Job drawing, mm, ordinate dimensions from the low corner. One solid piece. A direction names the side the tool comes from. Round coordinates to 2 decimals unless told otherwise and drop trailing zeros. Loops run counter-clockwise (first coordinate to the right, second up) from the corner with the lowest first, then second, coordinate; pieces in that order, holes last.
1) Mould opens along Z. For the marked faces 1, 2, 3 and 4 say: +Z half, -Z half, draft (parallel to the pull), parting line (faces both ways), or undercut.
2) Band-saw the part on B-B, the plane y = 5. Write the cut outline in (x, z), then the cut area to 3 significant figures.
3) Band-saw the part on C-C, the plane z = 2.25. Write the cut outline in (x, y).
4) Probe line 1 (Y direction, x = 7.5, z = 0.9); line 2 (X direction, y = 7, z = 12.25). List the from-to ranges inside material, lowest first.
5) Drop flat-ended pins along their axis: P1, Ø2, axis at y = 7.5, z = 5, coming from the +X side; P2, Ø2.5, axis at y = 5, z = 7.5, coming from the -X side. Give the stop position or say it passes through.
6) 3-axis set-ups, long thin cutter, end or side, ignore diameter. For the marked faces 5 and 6: which of +Z, -Z, +X, -X, +Y, -Y reach the whole face in a straight line?
7) Band-saw the part on D-D, the plane y = 9. Write the cut outline in (x, z), then the cut area to 3 significant figures.
8) Band-saw the part on A-A, the plane z = 7.5. Write the cut outline in (x, y), then the cut area to 3 significant figures.
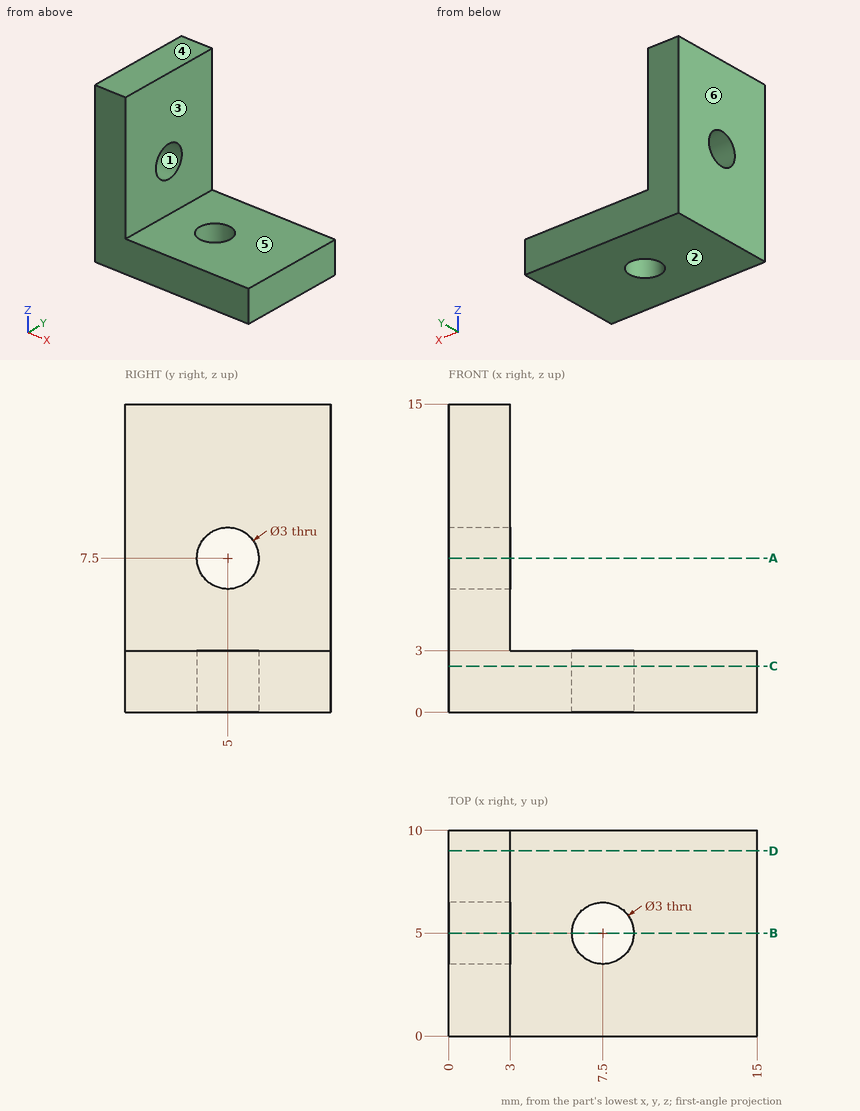
Reported:
1. face 1: undercut
1. face 2: -Z half
1. face 3: draft
1. face 4: +Z half
2. outline: (0, 0) - (6, 0) - (6, 3) - (3, 3) - (3, 6) - (0, 6) - close; (0, 9) - (3, 9) - (3, 15) - (0, 15) - close; (9, 0) - (15, 0) - (15, 3) - (9, 3) - close
2. area: 63.0 mm2
3. outline: (0, 0) - (15, 0) - (15, 10) - (0, 10) - close; hole circle Ø3 at (7.5, 5)
4. line 1: y = 0 to 3.5, 6.5 to 10
4. line 2: x = 0 to 3
5. P1: stops at x = 3
5. P2: passes through
6. face 5: +Z, +X, +Y, -Y
6. face 6: +Z, -Z, -X, +Y, -Y
7. outline: (0, 0) - (15, 0) - (15, 3) - (3, 3) - (3, 15) - (0, 15) - close
7. area: 81.0 mm2
8. outline: (0, 0) - (3, 0) - (3, 3.5) - (0, 3.5) - close; (0, 6.5) - (3, 6.5) - (3, 10) - (0, 10) - close
8. area: 21.0 mm2
